```python
from build123d import *

# Parameters (mm, degrees)
SKETCH1_W           = 43.3
SKETCH1_H           = 43.3
SKETCH1_R           = 1.45
BOSS_EXTRUDE1_DEPTH = 1.5
BOSS_EXTRUDE2_DEPTH = 2.5
SKETCH3_W           = 30.8
SKETCH3_H           = 8
BOSS_EXTRUDE3_DEPTH = 10
SKETCH4_W           = 23.5
SKETCH4_H           = 15.7
BOSS_EXTRUDE4_DEPTH = 25


with BuildPart() as part:
    # Sketch1 → Boss-Extrude1 (new body)
    with BuildSketch(Plane(origin=(0, 0, 0), x_dir=(1, 0, 0), z_dir=(0, 1, 0))):
        with Locations((21.65, 21.65)):
            Rectangle(SKETCH1_W, SKETCH1_H)
        with Locations(Location((3.2, 3.2, 0), (0, 0, 270))):
            Circle(SKETCH1_R, mode=Mode.SUBTRACT)
        with Locations(Location((3.2, 40.1, 0), (0, 0, 270))):
            Circle(SKETCH1_R, mode=Mode.SUBTRACT)
        with Locations(Location((40.1, 40.1, 0), (0, 0, 270))):
            Circle(SKETCH1_R, mode=Mode.SUBTRACT)
        with Locations(Location((40.1, 3.2, 0), (0, 0, 270))):
            Circle(SKETCH1_R, mode=Mode.SUBTRACT)
    extrude(amount=BOSS_EXTRUDE1_DEPTH)

    # Sketch2 → Boss-Extrude2 (add)
    with BuildSketch(Plane.XZ):
        Polygon((0, -35.9), (0, -7.4), (7.4, -7.4), (7.4, 0), (35.9, 0), (35.9, -7.4), (43.3, -7.4), (43.3, -35.9), (35.9, -35.9), (35.9, -43.3), (7.4, -43.3), (7.4, -35.9), align=None)
    extrude(amount=BOSS_EXTRUDE2_DEPTH)

    # Sketch3 → Boss-Extrude3 (add)
    with BuildSketch(Plane(origin=(0, 1.5, 0), x_dir=(1, 0, 0), z_dir=(0, 1, 0))):
        with Locations((21.9, 4)):
            Rectangle(SKETCH3_W, SKETCH3_H)
    extrude(amount=BOSS_EXTRUDE3_DEPTH)

    # Sketch4 → Boss-Extrude4 (add)
    with BuildSketch(Plane(origin=(0, 1.5, 0), x_dir=(1, 0, 0), z_dir=(0, 1, 0))):
        with Locations((21.65, 35.45)):
            Rectangle(SKETCH4_W, SKETCH4_H)
    extrude(amount=BOSS_EXTRUDE4_DEPTH)


solid = part.part
```
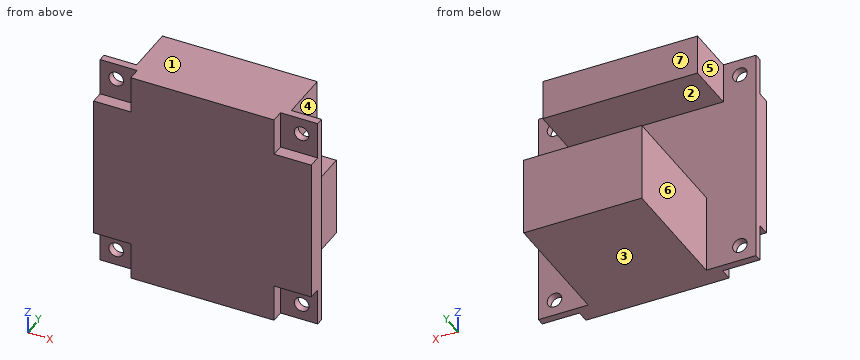
The model under review builds one solid part; all positions refer to its coordinate system, in mm. Face numbers are marked on the shaded views. A direction names the side the tool comes from. Coordinates: 2 decimals unless noted, no trailing zeros. Write each loop counter-clockwise with the first axis right and the second up, starting at its lowest first coordinate (ties: lowest second). Pieces come first, ordered by that corner, then holes.
1) We need section A-A on z = -3.2. State the section outline as (x, y) points, then the cut area to 4 significant figures.
2) To check wall thickness, follow probe 1 along X at (y, z) = (0.95, -3.2); probe 2 along Z at (x, y) = (15.5, 7.25); probe 3 along Y at (x, z) = (3, -13.5). State the ranges of each line that lie inside material, in increasing order.
3) Clearance check with flat-ended pins moving along their axes: pin 1 Ø9 at (y, z) = (6.5, -5) entering from -X; pin 2 Ø5 at (y, z) = (2.5, -22.5) entering from -X; pin 3 Ø8 at (y, z) = (15, -32) entering from -X; pin 4 Ø9 at (x, z) = (23, -3.5) entering from +Y. State where each tip first meets the part, or that it passes through.
4) Machinability: for the marked faces 5, 6 and 7, which of the approach directions +Z, -Z, +X, -X, +Y, -Y give a long, thin tool a straight path to every point of the face, cutting with its end or side? Answer none if there is none.
5) We need section C-C on y = 2.5. State the section outline as (x, z) points.
6) We need section B-B on x = 3.2. State the section outline as (y, z) points, then the cut area to 4 significant figures.
7) We need section D-D on z = -29. State the section outline as (x, y) points.
8) The part is to be moulded in two halves that separate along Z. For the marked faces 1, 2, 3 and 4, say which applies: pulls with the +Z half, pulls with the -Z half, needs draft (parallel to the pull), parting line crosses it, or undercut.
Answer list:
1. outline: (0, 0) - (1.75, 0) - (1.75, 1.5) - (0, 1.5) - close; (4.65, 0) - (7.4, 0) - (7.4, -2.5) - (35.9, -2.5) - (35.9, 0) - (38.65, 0) - (38.65, 1.5) - (37.3, 1.5) - (37.3, 11.5) - (6.5, 11.5) - (6.5, 1.5) - (4.65, 1.5) - close; (41.55, 0) - (43.3, 0) - (43.3, 1.5) - (41.55, 1.5) - close
1. area: 435.5 mm2
2. probe 1: x = 0 to 1.75, 4.65 to 38.65, 41.55 to 43.3
2. probe 2: z = -43.3 to -27.6, -8 to 0
2. probe 3: y = -2.5 to 1.5
3. pin 1: stops at x = 6.5
3. pin 2: stops at x = 0
3. pin 3: stops at x = 9.9
3. pin 4: stops at y = 11.5
4. face 5: +Z, -Z, -X, +Y
4. face 6: -Z, -X, +Y
4. face 7: +Z, +X, -X, +Y
5. outline: (6.5, -8) - (37.3, -8) - (37.3, 0) - (6.5, 0) - close; (9.9, -43.3) - (33.4, -43.3) - (33.4, -27.6) - (9.9, -27.6) - close
6. outline: (-2.5, -35.9) - (0, -35.9) - (0, -38.65) - (1.5, -38.65) - (1.5, -4.65) - (0, -4.65) - (0, -7.4) - (-2.5, -7.4) - close; (0, -43.3) - (1.5, -43.3) - (1.5, -41.55) - (0, -41.55) - close; (0, -1.75) - (1.5, -1.75) - (1.5, 0) - (0, 0) - close
6. area: 127.5 mm2
7. outline: (0, -2.5) - (43.3, -2.5) - (43.3, 1.5) - (33.4, 1.5) - (33.4, 26.5) - (9.9, 26.5) - (9.9, 1.5) - (0, 1.5) - close
8. face 1: pulls with the +Z half
8. face 2: undercut
8. face 3: pulls with the -Z half
8. face 4: needs draft
